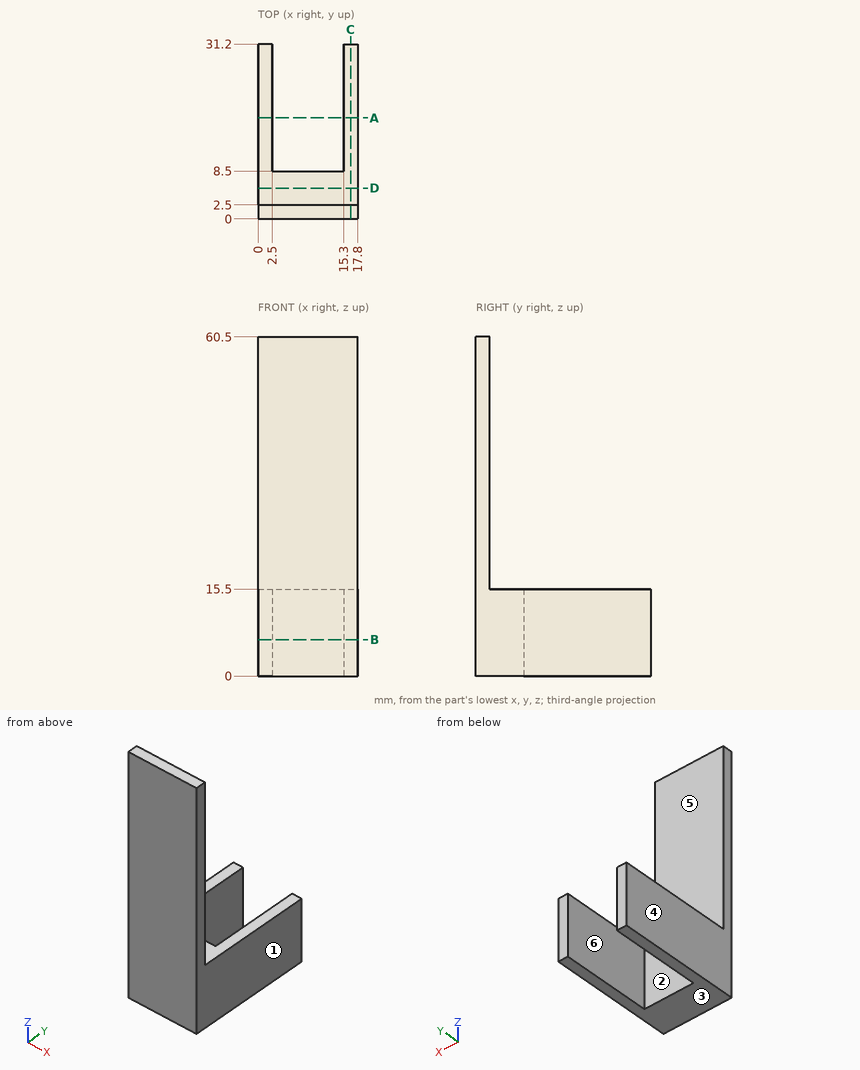
Design review of the part shown in the three views and the two pictorial views. Dimensions are in mm from the part's minimum x, y and z. A direction names the side the tool comes from. Round coordinates to 2 decimals unless told otherwise and drop trailing zeros. Order: outer loops, then holes, each group sorted by start corner. A loop starts at its lowest first (then second) coordinate and runs counter-clockwise, first axis right, second up.
(1) Take a section at B-B, the plane z = 6.5. State the section outline as (x, y) points, plus the area to 3 significant figures.
Working result:
outline: (0, 0) - (17.8, 0) - (17.8, 31.2) - (15.3, 31.2) - (15.3, 8.5) - (2.5, 8.5) - (2.5, 31.2) - (0, 31.2) - close
area: 265 mm2
(2) Take a section at D-D, the plane y = 5.5. State the section outline as (x, z) points, plus the area to 3 significant figures.
Working result:
outline: (0, 0) - (17.8, 0) - (17.8, 15.5) - (0, 15.5) - close
area: 276 mm2
(3) Wall thickness on L1, parallel to X at y = 29.5, z = 6; L2, parallel to Y at x = 15.25, z = 10; L3, parallel to Y at x = 15, z = 22: over which ranges is each line inside the solid? List them lowest first.
Working result:
L1: x = 0 to 2.5, 15.3 to 17.8
L2: y = 0 to 8.5
L3: y = 0 to 2.5
(4) Take a section at A-A, the plane y = 18. State the section outline as (x, z) points.
Working result:
outline: (0, 0) - (2.5, 0) - (2.5, 15.5) - (0, 15.5) - close; (15.3, 0) - (17.8, 0) - (17.8, 15.5) - (15.3, 15.5) - close
(5) Tool access review of the marked faces 4, 5 and 6: name each direction out of +Z, -Z, +X, -X, +Y, -Y from which nothing blocks a thin tool from reaching the whole face with its end or side.
Working result:
face 4: +Z, -Z, -X, +Y, -Y
face 5: +Z, +X, -X, +Y
face 6: +Z, -Z, +Y
(6) For P1, Ø10, axis at x = 11.5, z = 9, coming from the +Y side; P2, Ø4, axis at x = 7.5, z = 6.5, coming from the +Y side; P3, Ø9, axis at x = 10, z = 37, coming from the +Y side; P4, Ø4, axis at x = 13.5, y = 20, coming from the +Z side, all flat-tipped, find the tip position at first contact; note any pin that passes through.
Working result:
P1: stops at y = 31.2
P2: stops at y = 8.5
P3: stops at y = 2.5
P4: stops at z = 15.5
(7) Take a section at C-C, the plane x = 16.5. State the section outline as (y, z) points, plus the area to 3 significant figures.
Working result:
outline: (0, 0) - (31.2, 0) - (31.2, 15.5) - (2.5, 15.5) - (2.5, 60.5) - (0, 60.5) - close
area: 596 mm2
(8) Mouldability with a two-part tool opening along X and no side actions: class the marked faces 1, 2 and 3 as released by +X, released by -X, zero draft, split by the parting line, or undercut.
Working result:
face 1: released by +X
face 2: undercut
face 3: zero draft
